Autodesk Inventor part; units mm, degrees
ref_plane "YZ Plane" through (0, 0, 0) normal (1, 0, 0) x (0, 1, 0)
ref_plane "XZ Plane" through (0, 0, 0) normal (0, 1, 0) x (-1, 0, 0)
ref_plane "XY Plane" through (0, 0, 0) normal (0, 0, 1) x (1, 0, 0)
sketch "Schizzo1" plane through (0, 0, 0) normal (1, 0, 0) x (0, 1, 0)
  line L0 (10, 20) -> (-10, 20)
  line L1 (-10, 20) -> (-10, -20)
  line L2 (-10, -20) -> (10, -20)
  line L3 (10, -20) -> (10, 20)
  line L4 (0, 0) -> (10, 0) construction
  line L5 (0, 0) -> (0, -19.4896) construction
  circle A0 centre (0, 16) radius 2.5
  circle A1 centre (0, -16) radius 2.5
  circle A2 centre (5, 0) radius 2.5
  circle A3 centre (-5, 0) radius 2.5
  dimension "d0" = 40
  dimension "d1" = 20
  dimension "d2" = 4
  dimension "d3" = 5
  dimension "d8" = 5
  dimension "d9" = 5
  dimension "d10" = 5
  dimension "d11" = 10
extrude "Estrusione1" add sketch "Schizzo1" along normal mid plane 5 contours L3 L2 L1 L0 | A2 | A3
fillet "Raccordo1" radius 2 4 edges at (0, 10, 20) (0, -10, 20) (0, 10, -20) (0, -10, -20)
extrude "Estrusione2" cut sketch "Schizzo1" along normal mid plane 5 contours A2 | A3
properties part number "perno"
Check sheet for the modelled part. Datum: model origin and axes. Units: mm. Round coordinates to 2 decimals unless told otherwise and drop trailing zeros. Loops run counter-clockwise (first coordinate to the right, second up) from the corner with the lowest first, then second, coordinate; pieces in that order, holes last.
1. Sectioned sample at D-D on z = 16. Record the boundary of the cut face in (x, y), and give its area (3 significant figures).
2. Gauge pin test, flat end, axial feed: pin 1 Ø8 at (y, z) = (0, -16) entering from +X. Record the tip position at first contact, or that the pin passes through.
3. Scan lines: probe 1 along Z at (x, y) = (-1.15, 0); probe 2 along Z at (x, y) = (0.85, -5); probe 3 along Z at (x, y) = (1.2, -2.25). Record each from-to range of solid material in increasing order.
4. Sectioned sample at C-C on y = 0. Record the boundary of the cut face in (x, z).
5. Sectioned sample at B-B on y = 5. Record the boundary of the cut face in (x, z), and give its area (3 significant figures).
6. Mould release check, pull along Z, two halves, no side actions. Record for faces 1 (the cylindrical face through (-0.035, 7.385, -0.751)), 2 (the cylindrical face through (0.04, 9.43, 19.4)), 3 (the cylindrical face through (0.04, -0.54, -18.44)), 4 (the flat face through (-2.5, 0, 0)): released by +Z, released by -Z, zero draft, split by the parting line, or undercut.
7. Sectioned sample at A-A on z = 0. Record the boundary of the cut face in (x, y), and give its area (3 significant figures).
Recorded:
1. outline: (-2.5, -10) - (2.5, -10) - (2.5, -2.5) - (-2.5, -2.5) - close; (-2.5, 2.5) - (2.5, 2.5) - (2.5, 10) - (-2.5, 10) - close
1. area: 75.0 mm2
2. pin 1: stops at x = 2.5
3. probe 1: z = -20 to -18.5, -13.5 to 13.5, 18.5 to 20
3. probe 2: z = -20 to -2.5, 2.5 to 20
3. probe 3: z = -20 to -17.09, -14.91 to 14.91, 17.09 to 20
4. outline: (-2.5, -20) - (2.5, -20) - (2.5, -18.5) - (-2.5, -18.5) - close; (-2.5, -13.5) - (2.5, -13.5) - (2.5, 13.5) - (-2.5, 13.5) - close; (-2.5, 18.5) - (2.5, 18.5) - (2.5, 20) - (-2.5, 20) - close
5. outline: (-2.5, -20) - (2.5, -20) - (2.5, -2.5) - (-2.5, -2.5) - close; (-2.5, 2.5) - (2.5, 2.5) - (2.5, 20) - (-2.5, 20) - close
5. area: 175 mm2
6. face 1: undercut
6. face 2: released by +Z
6. face 3: undercut
6. face 4: zero draft
7. outline: (-2.5, -10) - (2.5, -10) - (2.5, -7.5) - (-2.5, -7.5) - close; (-2.5, -2.5) - (2.5, -2.5) - (2.5, 2.5) - (-2.5, 2.5) - close; (-2.5, 7.5) - (2.5, 7.5) - (2.5, 10) - (-2.5, 10) - close
7. area: 50.0 mm2
